Input: part model. Units: mm. Frame: model coordinates. A direction names the side the tool comes from. Coordinates: 2 decimals unless noted, no trailing zeros. Write each loop counter-clockwise with the first axis right and the second up, starting at its lowest first coordinate (ties: lowest second). Pieces come first, ordered by that corner, then holes. Notation, with made-up numbers: M -4.75,34.5 L 13.25,34.5 A25 cw 13.25,70.5 Z; hole C 9.5,74 d3. An arc over 180 degrees is marked long. Answer as a JSON object with one key per item and string values. Group by question number.
from build123d import *

# Parameters (mm, degrees)
F0_R     = 29.6
F0_R_2   = 9
F0_R_3   = 3.5
F1_DEPTH = 4
F0_R_4   = 1.65
F2_DEPTH = 8


with BuildPart() as f1:
    # F0 (on Top) → F1 (new body)
    with BuildSketch(Plane.XY):
        Circle(F0_R)
        Circle(F0_R_2, mode=Mode.SUBTRACT)
        Circle(F0_R_2)
        Circle(F0_R_3, mode=Mode.SUBTRACT)
    extrude(amount=F1_DEPTH)

    # F0 (on Top) → F2 (join)
    with BuildSketch(Plane.XY):
        Circle(F0_R_2)
        Circle(F0_R_3, mode=Mode.SUBTRACT)
        Circle(F0_R_3)
        Circle(F0_R_4, mode=Mode.SUBTRACT)
    extrude(amount=-F2_DEPTH)


solid = f1.part
Q1. Draft query along Y for faces 1 (the flat face through (1, -2, 0)), 2 (the flat face through (-7, -6, 0)), 3 (the cylindrical face through (-6.4, -28.9, 2)). Return one class per face: released by +Y, released by -Y, zero draft, split by the parting line, or undercut.
Q2. Access query for faces 4 (the flat face through (0, -6, 4)), 5 (the cylindrical face through (3.233, -1.341, 1.972)), 6 (the cylindrical face through (-1.172, 8.923, -3.944)). Directions: +Z, -Z, +X, -X, +Y, -Y. A direction counts if a zero-diameter tool reaches every point of the face in a straight line with its end or side. Return the directions, or none.
Q3. Section C-C, the plane z = -3. Return the cut outline in (x, y), and give its area (3 significant figures).
Q4. Section A-A, the plane y = 0. Return the cut outline in (x, z).
Q5. Pin query (flat end, axial travel): pin 1 Ø1.5 at (x, y) = (9, 17) entering from -Z; pin 2 Ø5.5 at (x, y) = (0, 0) entering from -Z; pin 3 Ø3 at (x, z) = (-21.5, -3) entering from +Y (3 decimals); pin 4 Ø6 at (x, z) = (13.5, 0.5) entering from +Y. Return the tip coordinate at first contact, or that it passes through.
Q6. Line query: line 1 (Y direction, x = 0, z = -1.5); line 2 (Y direction, x = 0, z = 1.7); line 3 (Z direction, x = 5, y = 13.5). Output: solid intervals per line, ascending. Write a range as from..to.
Q7. Section D-D, the plane y = -8. Return the cut outline in (x, z), and give its area (3 significant figures).
Filled in:
{
 "1": {"face 1": "undercut", "face 2": "zero draft", "face 3": "split by the parting line"},
 "2": {"face 4": "+Z, +X, -X, +Y, -Y", "face 5": "+Z", "face 6": "-Z"},
 "3": {"outline": "C 0,0 d18; hole C 0,0 d3.3", "area": "246 mm^2"},
 "4": {"outline": "M -29.6,0 L -9,0 L -9,-8 L -1.65,-8 L -1.65,0 L -3.5,0 L -3.5,4 L -29.6,4 Z; M 1.65,-8 L 9,-8 L 9,0 L 29.6,0 L 29.6,4 L 3.5,4 L 3.5,0 L 1.65,0 Z"},
 "5": {"pin 1": "z = 0", "pin 2": "z = -8", "pin 3": "through", "pin 4": "y = 27.68"},
 "6": {"line 1": "-9..-1.65, 1.65..9", "line 2": "-29.6..-3.5, 3.5..29.6", "line 3": "0..4"},
 "7": {"outline": "M -28.5,0 L -4.12,0 L -4.12,-8 L 4.12,-8 L 4.12,0 L 28.5,0 L 28.5,4 L -28.5,4 Z", "area": "294 mm^2"}
}
